```python
from build123d import *

# Parameters (mm, degrees)
SKETCH2_R               = 2.5
CUT_EXTRUDE1_DEPTH      = 39
SKETCH3_R               = 3
CUT_EXTRUDE2_DEPTH      = 26
CUT_EXTRUDE2_DEPTH_BACK = 26


with BuildPart() as part:
    # Sketch1 → Revolve1 (revolve)
    with BuildSketch(Plane.XY):
        Polygon((0, 30.794117647), (25, 30.794117647), (25, 25.794117647), (14, 25.794117647), (14, -2.205882353), (25, -2.205882353), (25, -7.205882353), (0, -7.205882353), align=None)
    revolve(axis=Axis((0, -19.166666667, 0), (0, 1, 0)))

    # Sketch2 → Cut-Extrude1 (cut, through all)
    with BuildSketch(Plane(origin=(0, 30.794117647, 0), x_dir=(1, 0, 0), z_dir=(0, 1, 0))):
        with Locations((12.727922061, 12.727922061)):
            Circle(SKETCH2_R)
        with Locations((12.727922061, -12.727922061)):
            Circle(SKETCH2_R)
        with Locations((-12.727922061, -12.727922061)):
            Circle(SKETCH2_R)
        with Locations((-12.727922061, 12.727922061)):
            Circle(SKETCH2_R)
        with BuildLine():
            Line((-2.5, 7.599342077), (-2.5, 10.5))
            Line((-2.5, 10.5), (2.5, 10.5))
            Line((2.5, 10.5), (2.5, 7.599342077))
            ThreePointArc((2.5, 7.599342077), (0, -8), (-2.5, 7.599342077))
        make_face()
    extrude(amount=-CUT_EXTRUDE1_DEPTH, mode=Mode.SUBTRACT)

    # Sketch3 → Cut-Extrude2 (cut, two sides)
    with BuildSketch(Plane(origin=(0, 0, 0), x_dir=(0, 0, -1), z_dir=(1, 0, 0))) as cut_extrude2_sk:
        with Locations((0, 11.794117647)):
            Circle(SKETCH3_R)
    extrude(amount=CUT_EXTRUDE2_DEPTH, mode=Mode.SUBTRACT)
    extrude(cut_extrude2_sk.sketch, amount=-CUT_EXTRUDE2_DEPTH_BACK, mode=Mode.SUBTRACT)


solid = part.part
```
Read the model definition and answer for the solid it produces. Units are mm, in the model's axes. A direction names the side the tool comes from. Give positions to 0.01 mm unless a question says otherwise; leave off trailing zeros. Loops run counter-clockwise (first coordinate to the right, second up) from the corner with the lowest first, then second, coordinate; pieces in that order, holes last.
Item 1: The part is cut by section D-D (y = -1.5). Write down the section's boundary in (x, z), and give its area (3 significant figures).
Item 2: For faces 1 (the flat face through (0, 12, -10.5)), 2 (the flat face through (-6, -7.206, -6)), 3 (the flat face through (10.8, 25.794, 10.8)), determine the directions among +Z, -Z, +X, -X, +Y, -Y from which every point of the face is accessible in a straight line to the end or side of a thin tool.
Item 3: The mould has two halves that part along Y. Classify faces 4 (the flat face through (6, 30.794, -6)), 5 (the cylindrical face through (-10.7, 11.9, 3)), 6 (the cylindrical face through (-10.343, 28.329, 11.977)): released by +Y, released by -Y, zero draft, split by the parting line, or undercut.
Item 4: Find the intervals of material crossed by line 1 along Y through (x, z) = (-3.5, -18.5); line 2 along X through (y, z) = (-3, -13); line 3 along Y through (x, z) = (10, 0), in increasing order.
Item 5: The part is cut by section C-C (x = -12.5). Give the number of separate pieces and of enclosed holes in the cut face, and give its area (3 significant figures).
Item 6: Each of these flat-tipped pins is pushed along its axis until it touches: pin 1 Ø0.9 at (y, z) = (20, -9.5) entering from -X; pin 2 Ø7 at (y, z) = (11.79, 0) entering from +X; pin 3 Ø3 at (y, z) = (3, 14) entering from -X. Where does it stop, or does it pass through?
Item 7: The part is cut by section A-A (x = 0). Write down the section's boundary in (y, z).
Item 8: The part is cut by section B-B (z = 0). Write down the section's boundary in (x, y).
Taken from the geometry:
1. outline: circle Ø28 at (0, 0); hole (-2.5, -10.5) - (2.5, -10.5) - (2.5, -7.6) arc R8 ccw (long way) to (-2.5, -7.6) - close
1. area: 402 mm2
2. face 1: +Y, -Y
2. face 2: +Z, -Z, +X, -X, -Y
2. face 3: none
3. face 4: released by +Y
3. face 5: undercut
3. face 6: zero draft
4. line 1: y = -7.21 to -2.21, 25.79 to 30.79
4. line 2: x = -21.35 to -15.21, -10.24 to 10.24, 15.21 to 21.35
4. line 3: y = -7.21 to 8.79, 14.79 to 30.79
5. separate pieces: 5
5. enclosed holes: 1
5. area: 658 mm2
6. pin 1: stops at x = -10.68
6. pin 2: stops at x = 14
6. pin 3: stops at x = -6.3
7. outline: (-7.21, -25) - (-2.21, -25) - (-2.21, -14) - (25.79, -14) - (25.79, -25) - (30.79, -25) - (30.79, -10.5) - (-7.21, -10.5) - close; (-7.21, 8) - (30.79, 8) - (30.79, 25) - (25.79, 25) - (25.79, 14) - (-2.21, 14) - (-2.21, 25) - (-7.21, 25) - close
8. outline: (-25, -7.21) - (-8, -7.21) - (-8, 8.79) - (-14, 8.79) - (-14, -2.21) - (-25, -2.21) - close; (-25, 25.79) - (-14, 25.79) - (-14, 14.79) - (-8, 14.79) - (-8, 30.79) - (-25, 30.79) - close; (8, -7.21) - (25, -7.21) - (25, -2.21) - (14, -2.21) - (14, 8.79) - (8, 8.79) - close; (8, 14.79) - (14, 14.79) - (14, 25.79) - (25, 25.79) - (25, 30.79) - (8, 30.79) - close
